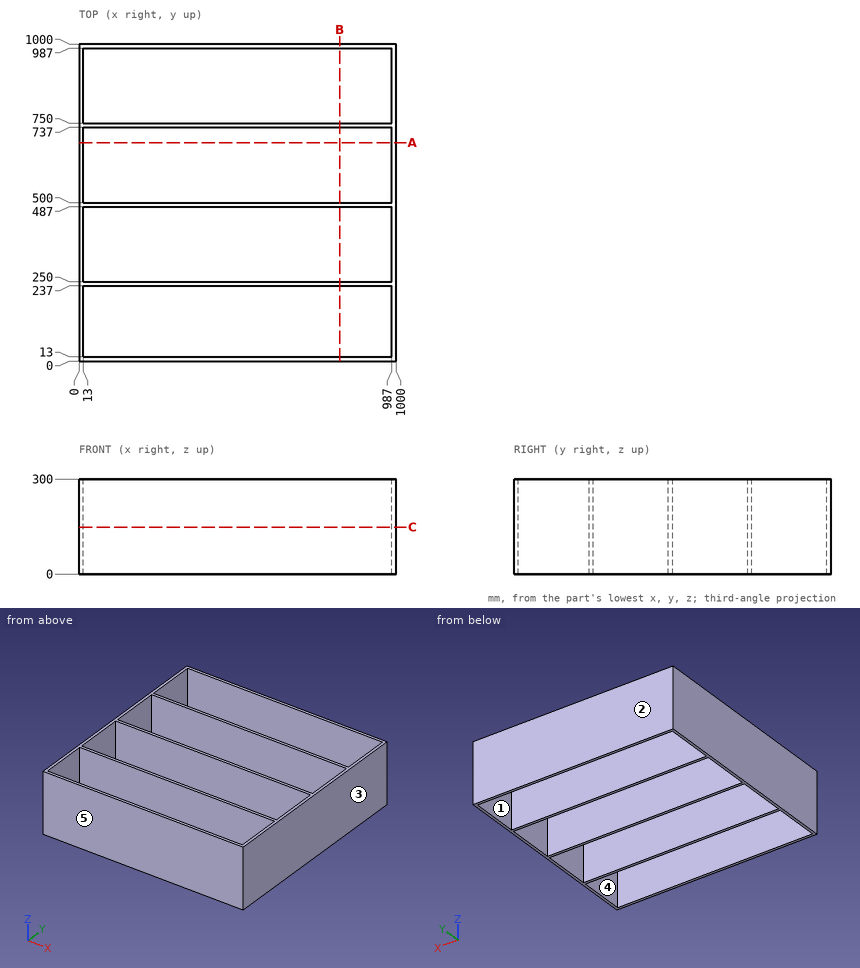
The figure shows three views and two pictorial views of one solid part (mm, origin at its lowest corner). Answer the questions. A direction names the side the tool comes from. Round coordinates to 2 decimals unless told otherwise and drop trailing zeros. Order: outer loops, then holes, each group sorted by start corner. A loop starts at its lowest first (then second) coordinate and runs counter-clockwise, first axis right, second up.
Q1. Find the intervals of material crossed by line 1 along Y through (x, z) = (95.5, 133.5); line 2 along X through (y, z) = (581, 59.5), in increasing order.
Solution:
line 1: y = 0 to 13, 237 to 250, 487 to 500, 737 to 750, 987 to 1000
line 2: x = 0 to 13, 987 to 1000
Q2. A tool of negligible diameter and unlimited length cuts with its end or side. For the marked faces 1 and 2, from which of +Z, -Z, +X, -X, +Y, -Y can it reach the whole face along a straight path? Write none if from no direction.
Solution:
face 1: +Z, -Z
face 2: +Z, -Z, +X, -X, +Y
Q3. A cutting plane is placed at A-A, the plane y = 689. Determine the outline of the cut face in (x, z).
Solution:
outline: (0, 0) - (13, 0) - (13, 300) - (0, 300) - close; (987, 0) - (1000, 0) - (1000, 300) - (987, 300) - close
Q4. Given pin 1 Ø3 at (x, z) = (652, 127.5) entering from -Y, flat-ended and moving along its own axis, determine where the tip first touches the part or whether it passes through.
Solution:
pin 1: stops at y = 0
Q5. A cutting plane is placed at B-B, the plane x = 822. Determine the outline of the cut face in (y, z).
Solution:
outline: (0, 0) - (13, 0) - (13, 300) - (0, 300) - close; (237, 0) - (250, 0) - (250, 300) - (237, 300) - close; (487, 0) - (500, 0) - (500, 300) - (487, 300) - close; (737, 0) - (750, 0) - (750, 300) - (737, 300) - close; (987, 0) - (1000, 0) - (1000, 300) - (987, 300) - close
Q6. A cutting plane is placed at C-C, the plane z = 148.5. Determine the outline of the cut face in (x, y).
Solution:
outline: (0, 0) - (1000, 0) - (1000, 1000) - (0, 1000) - close; hole (13, 13) - (987, 13) - (987, 237) - (13, 237) - close; hole (13, 250) - (987, 250) - (987, 487) - (13, 487) - close; hole (13, 500) - (987, 500) - (987, 737) - (13, 737) - close; hole (13, 750) - (987, 750) - (987, 987) - (13, 987) - close
Q7. The mould has two halves that part along X. Classify the marked faces 3, 4 and 5: pulls with the +X half, pulls with the -X half, needs draft (parallel to the pull), parting line crosses it, or undercut.
Solution:
face 3: pulls with the +X half
face 4: undercut
face 5: needs draft
